Autodesk Inventor part; units mm, degrees
ref_plane "Work Plane2" through (0, 4, 0) normal (0, 1, 0) x (-1, 0, 0)
ref_plane "YZ Plane" through (0, 0, 0) normal (1, 0, 0) x (0, 1, 0)
ref_plane "XY Plane" through (0, 0, 0) normal (0, 0, 1) x (1, 0, 0)
sketch "Sketch1" plane through (0, 0, 0) normal (1, 0, 0) x (0, 1, 0)
  circle A0 centre (0, 0) radius 2
  dimension "d0" = 4
extrude "Extrusion1" add sketch "Sketch1" along normal blind 7.5
ref_plane "Work Plane1" through (0, 2, 0) normal (0, 1, 0) x (-1, 0, 0)
sketch "Sketch2" plane through (0, 2, 0) normal (0, 1, 0) x (-1, 0, 0)
  arc A0 (14.5, 14.5) -> (14.5, -14.5) centre (14.5, 0) ccw
  arc A1 (14.5, 15.5) -> (14.5, -15.5) centre (14.5, 0) ccw
  line L0 (14.5, 15.5) -> (14.5, 14.5)
  line L1 (14.5, -14.5) -> (14.5, -15.5)
  point P0 (0, 0)
  dimension "d5" = 31
extrude "Extrusion2" add sketch "Sketch2" against normal blind 4
sketch "Sketch3" plane through (0, 2, 0) normal (0, 1, 0) x (1, 0, 0)
  point P0 (-14.5, -14.5)
  point P1 (-14.5, 14.5)
  point P2 (-14.5, 0)
  point P3 (-14.5, -15.5)
ref_plane "Work Plane2" through (0, 4, 0) normal (0, 1, 0) x (-1, 0, 0)
sketch "Sketch4" plane through (0, 4, 0) normal (0, 1, 0) x (-1, 0, 0)
  arc A0 (14.5, 15.5) -> (-1, 0) centre (14.5, 0) ccw
  arc A1 (14.5, 15.5) -> (14.5, -15.5) centre (14.5, 0) ccw
  arc A2 (14.5, 14.5) -> (14.5, -14.5) centre (14.5, 0) ccw
  line L0 (14.5, 15.5) -> (14.5, 14.5)
  arc A3 (14.5, 14.5) -> (14.5, -14.5) centre (14.5, 0) ccw
  line L1 (14.5, -14.5) -> (14.5, -15.5)
  line L2 (14.5, 14.5) -> (17.5, 14.5)
  line L3 (17.5, 14.5) -> (17.5, 15.5)
  line L4 (17.5, 15.5) -> (14.5, 15.5)
  line L5 (14.5, -15.5) -> (17.5, -15.5)
  line L6 (17.5, -15.5) -> (17.5, -14.5)
  line L7 (17.5, -14.5) -> (14.5, -14.5)
  point P0 (0, 0)
  dimension "d10" = 3
  dimension "d11" = 1
  dimension "d12" = 3
extrude "Extrusion3" add sketch "Sketch4" against normal blind 8
sketch "Sketch5" plane through (-17.5, 4, 15.5) normal (0, 0, 1) x (1, 0, 0)
  line L0 (3, 0) -> (3, -8)
  circle A0 centre (3, -4) radius 2.5
  line L1 (3, -8) -> (18.5, -8)
  line L2 (3, -6.5) -> (18.5, -8)
  line L3 (18.5, -8) -> (-0.017, -8)
  line L4 (-0.017, -8) -> (-0.017, 0)
  line L5 (-0.017, 0) -> (18.5, 0)
  line L6 (18.5, 0) -> (18.5, -8)
  line L7 (18.5, 0) -> (3, -1.5)
  point P0 (17.5, -4)
  dimension "d15" = 5
extrude "Extrusion4" cut sketch "Sketch5" against normal through all contours L5 L7 L0 | L0 A0 L3 L4 L5 | L2 L1 L0
sketch "Sketch6" plane through (-14.5, 0, -15.5) normal (0, 0, -1) x (-1, 0, 0)
  line L0 (0, 2.5) -> (0, -2.5)
  circle A0 centre (0, 0) radius 1
  point P0 (-14.5, 0)
  dimension "d18" = 2
extrude "Extrusion5" cut sketch "Sketch6" against normal through all
properties part number "Sujetador Espejo"
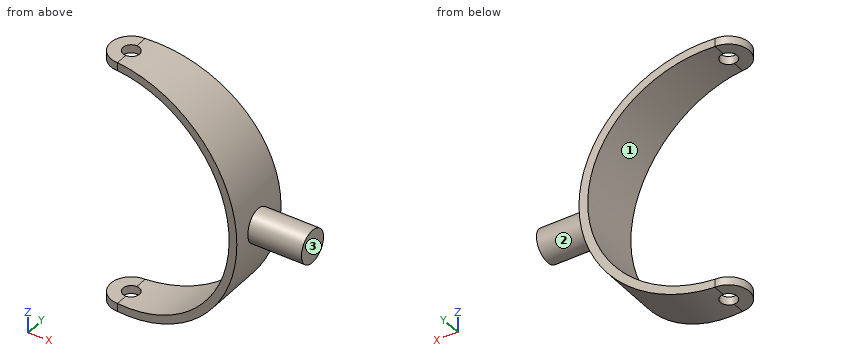
Here's how the part is built. I have some questions about the finished solid (model axes, mm). Face numbers are marked on the shaded views. Coordinates: 2 decimals unless noted, no trailing zeros. Loops run counter-clockwise (first coordinate to the right, second up) from the corner with the lowest first, then second, coordinate; pieces in that order, holes last. Notation, with made-up numbers: (1.25, 79.25) -> (38.25, 79.25) arc R23 ccw to (38.25, 94.25) -> close; hole circle Ø11 at (64.5, 38.5). An arc over 180 degrees is marked (long way). Use one line per item in the form item = value. Start each with the question number.
(1) If we section it at A-A (x = -1.5): Please give me the cut outline in (y, z).
(2) We'd pull the mould along Z, two halves only. Please class the marked faces 1, 2 and 3: pulls with the +Z half, pulls with the -Z half, needs draft (parallel to the pull), parting line crosses it, or undercut.
(3) Will these pins go through, and if not, where does the flat tip stop? pin 1 (2 mm diameter, centred on x = -4.5, z = 10.5, fed in from +Y); pin 2 (2 mm diameter, centred on x = -8, y = 0, fed in from -Z); pin 3 (1 mm diameter, centred on y = 0.5, z = -2, fed in from -X).
(4) If we section it at C-C (z = 0): Please give me the cut outline in (x, y).
(5) If we section it at D-D (y = 3.25): Please give me the cut outline in (x, z).
(6) Please list where these lines run through material, in increasing order: line 1 along Y through (x, z) = (-14.5, 14.7); line 2 along Z through (x, y) = (-14, 1); line 3 along Z through (x, y) = (-2.5, -2.5).
Verdict:
q1.outline = (-3.76, -8.44) -> (3.76, -8.44) -> (3.76, -6.42) -> (-3.76, -6.42) -> close; (-3.76, 6.42) -> (3.76, 6.42) -> (3.76, 8.44) -> (-3.76, 8.44) -> close
q2.face_1 = undercut
q2.face_2 = parting line crosses it
q2.face_3 = needs draft
q3.pin_1 = 3.56
q3.pin_2 = -14.49
q3.pin_3 = -0.22
q4.outline = (0, -3.9) -> (1, -4) -> (1, -2) -> (7.5, -2) -> (7.5, 2) -> (1, 2) -> (1, 4) -> (0, 3.9) -> close
q5.outline = (-6.75, -13.42) arc R15.5 ccw to (-6.75, 13.42) -> (-6.75, 12.26) arc R14.5 cw to (-6.75, -12.26) -> close
q6.line_1 = -2.5 to -1, 1 to 2.5
q6.line_2 = -15.49 to -14.49, 14.49 to 15.49
q6.line_3 = -9.81 to -8.14, 8.14 to 9.81
